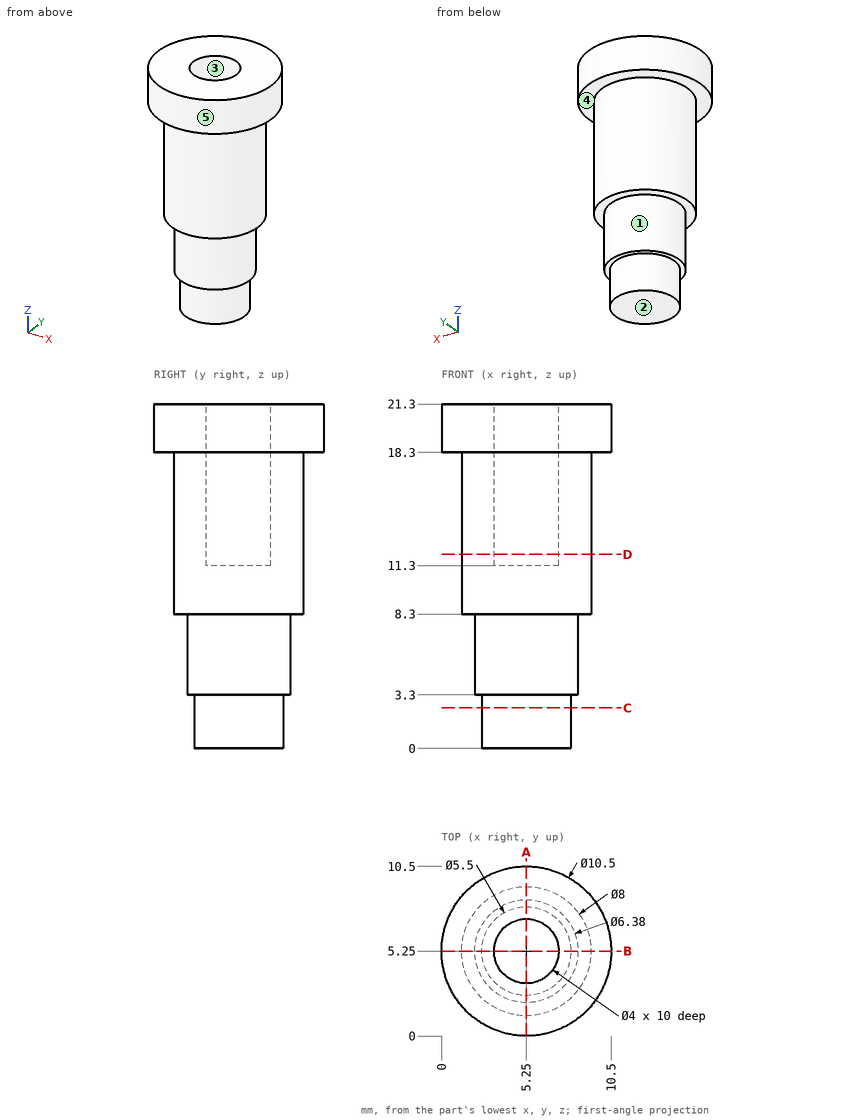
Here's the drawing with two shaded views (mm, measured from the low corner). I have some questions. A direction names the side the tool comes from. Round coordinates to 2 decimals unless told otherwise and drop trailing zeros. Order: outer loops, then holes, each group sorted by start corner. A loop starts at its lowest first (then second) coordinate and runs counter-clockwise, first axis right, second up. Notation, with made-up numbers: M 16.5,-4 L 46.5,-4 A14 ccw 46.5,2 Z; hole C 3.5,6.5 d1. An arc over 180 degrees is marked long. Use CSV: the item, a comma, the result in double quotes.
1) I need wall thicknesses on line 1 along X through (y, z) = (5.25, 14.25); line 2 along Z through (x, y) = (7, 4.5); line 3 along X through (y, z) = (3.5, 19.25). Which ranges of each line are inside material? Lowest first, please. Write a range as [from, to].
Taken from the geometry:
line 1,"[1.25, 3.25], [7.25, 9.25]"
line 2,"[0, 11.3]"
line 3,"[0.3, 4.28], [6.22, 10.2]"
2) I want a section at D-D (z = 12). List the corners of the cut face in (x, y) for me, then the cut area to 3 significant figures.
Taken from the geometry:
outline,"C 5.25,5.25 d8; hole C 5.25,5.25 d4"
area,"37.7 mm^2"
3) If we mould it in two halves opening along X, with no side actions, what happens to the marked faces 3, 4 and 5? For each: pulls with the +X half, pulls with the -X half, needs draft (parallel to the pull), parting line crosses it, or undercut.
Taken from the geometry:
face 3,"undercut"
face 4,"needs draft"
face 5,"parting line crosses it"
4) I want a section at C-C (z = 2.5). List the corners of the cut face in (x, y) for me.
Taken from the geometry:
outline,"C 5.25,5.25 d5.5"
5) I'm going to push flat-ended pins straight in: P1, Ø5, axis at x = 1.5, y = 5.5, coming from the -Z side; P2, Ø2, axis at y = 3.5, z = 3, coming from the +X side; P3, Ø3, axis at x = 6, z = 3.5, coming from the +Y side. Where does each tip first touch, or does it pass through?
Taken from the geometry:
P1,"z = 0"
P2,"x = 8.34"
P3,"y = 8.44"
6) I want a section at A-A (x = 5.25). List the corners of the cut face in (y, z) for me, then the cut area to 3 significant figures.
Taken from the geometry:
outline,"M 0,18.3 L 1.25,18.3 L 1.25,8.3 L 2.06,8.3 L 2.06,3.3 L 2.5,3.3 L 2.5,0 L 8,0 L 8,3.3 L 8.44,3.3 L 8.44,8.3 L 9.25,8.3 L 9.25,18.3 L 10.5,18.3 L 10.5,21.3 L 7.25,21.3 L 7.25,11.3 L 3.25,11.3 L 3.25,21.3 L 0,21.3 Z"
area,"122 mm^2"
7) On a 3-axis mill with a long thin cutter (end or side, diameter ignored), from which of +Z, -Z, +X, -X, +Y, -Y can I reach the whole of each face in a straight line? I mean the marked faces 1 and 2. Say none if no direction works.
Taken from the geometry:
face 1,"-Z"
face 2,"-Z, +X, -X, +Y, -Y"
